Check sheet for the drawn part. Datum: minimum x, y, z corner. Units: mm. A direction names the side the tool comes from. Give positions to 0.01 mm unless a question says otherwise; leave off trailing zeros. Order: outer loops, then holes, each group sorted by start corner. A loop starts at its lowest first (then second) coordinate and runs counter-clockwise, first axis right, second up. Notation, with made-up numbers: (22, 46.25) -> (70, 46.25) arc R16 cw to (70, 56.25) -> close; hole circle Ø7 at (-22.5, 65). An arc over 180 degrees is marked (long way). One line per question, with ' | ' between items. Start each with the question number.
Q1. Access from +Z, -Z, +X, -X, +Y, -Y to the whole of each face (thin tool, end or side, straight path). Record for the marked faces 4, 5, 6 and 7.
Q2. Section check B-B on y = 13.5. Give the number of separate pieces and of enclosed holes in the cut face, plus the area to 3 significant figures.
Q3. Go/stop test with flat-tipped pins: pin 1 (1.5 mm diameter, centred on x = 4, y = 21, fed in from +Z); pin 2 (7.5 mm diameter, centred on x = 16.66, y = 19.05, fed in from +Z); pin 3 (18 mm diameter, centred on x = 23.5, z = 17, fed in from +Y); pin 4 (5 mm diameter, centred on x = 18.5, y = 32, fed in from +Z). Record where each tip stops, or that it passes through.
Q4. Material ranges on probe 1 along X at (y, z) = (1, 19) (1 decimal); probe 2 along X at (y, z) = (19.05, 22.5) (1 decimal); probe 3 along Z at (x, y) = (12, 12), recorded low to high. Write a range as [from, to].
Q5. Mould release check, pull along Z, two halves, no side actions. Record for the marked faces 1, 2 and 3: released by +Z, released by -Z, zero draft, split by the parting line, or undercut.
Q6. Section check A-A on x = 29.5. Record the cut outline in (y, z).
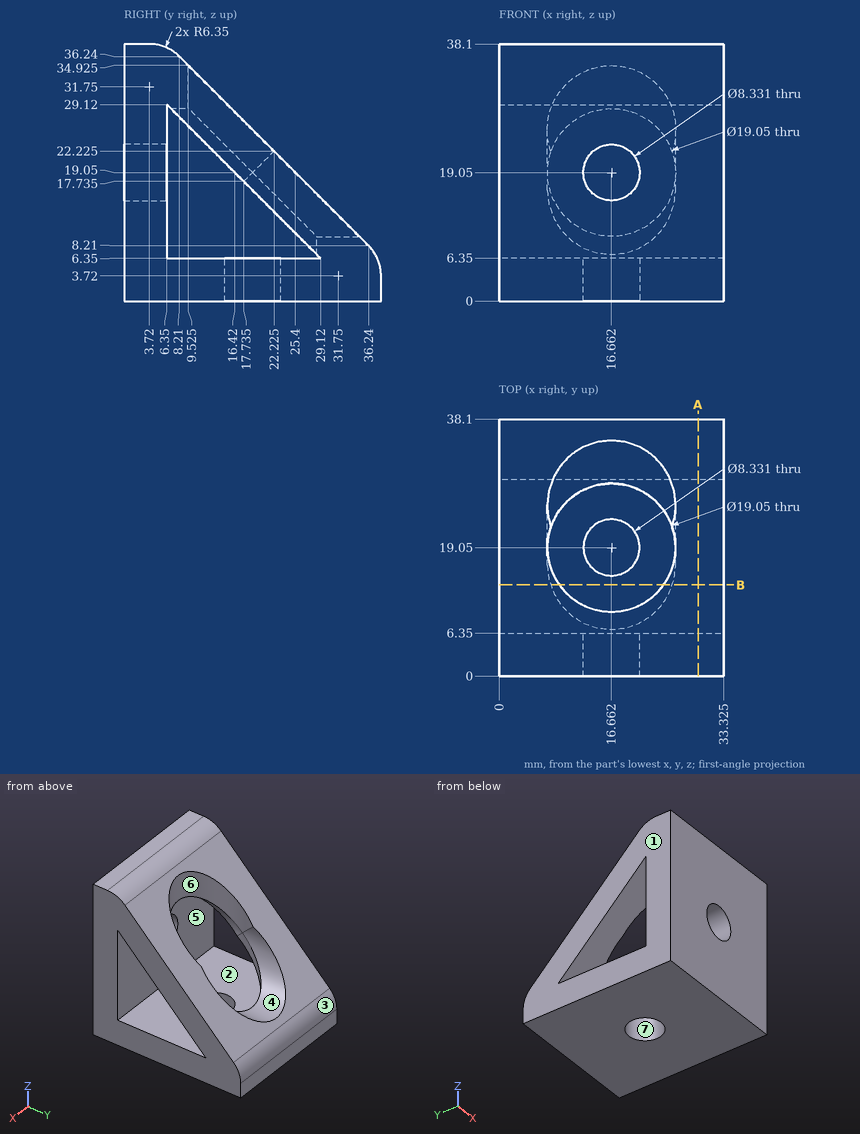
Filled in:
1) face 4: +Y | face 5: +X, -X | face 6: +Z | face 7: +Z, -Z
2) separate pieces: 3 | enclosed holes: 0 | area: 368 mm²
3) pin 1: z = 24.2 | pin 2: through | pin 3: y = 36.44 | pin 4: z = 10.57
4) probe 1: [0, 12.5], [20.8, 33.3] | probe 2: [0, 7.1], [26.2, 33.3] | probe 3: [0, 6.35]
5) face 1: zero draft | face 2: undercut | face 3: released by +Z
6) outline: (0, 0) -> (38.1, 0) -> (38.1, 3.72) arc R6.35 ccw to (36.24, 8.21) -> (8.21, 36.24) arc R6.35 ccw to (3.72, 38.1) -> (0, 38.1) -> close; hole (6.35, 6.35) -> (29.12, 6.35) -> (6.35, 29.12) -> close
